from build123d import *
from OCP.BRepFilletAPI import BRepFilletAPI_MakeChamfer

# Parameters (mm, degrees)
SKETCH1_W                = 13.2
SKETCH1_H                = 8
BOSS_EXTRUDE1_DEPTH      = 2
CUT_EXTRUDE1_DEPTH       = 12.914696807
CUT_EXTRUDE1_DEPTH_BACK  = 12.914696807
SKETCH3_W                = 2
SKETCH3_H                = 8
BOSS_EXTRUDE2_DEPTH      = 3.65
BOSS_EXTRUDE3_DEPTH      = 2
BOSS_EXTRUDE4_DEPTH      = 1.25
BOSS_EXTRUDE5_DEPTH      = 2.1
BOSS_EXTRUDE6_DEPTH      = 2.25
CHAMFER3_SIZE            = 1.5
CHAMFER4_SIZE            = 0.3
CHAMFER3_OF_MIRROR1_SIZE = 1.5
CHAMFER4_OF_MIRROR1_SIZE = 0.3
CUT_EXTRUDE2_DEPTH       = 15.141428499
CUT_EXTRUDE2_DEPTH_BACK  = 15.141428499
SKETCH10_W               = 1
SKETCH10_H               = 8
CUT_EXTRUDE3_DEPTH       = 15.418477728
CUT_EXTRUDE3_DEPTH_BACK  = 1
SKETCH12_W               = 6
SKETCH12_H               = 3.8
CUT_EXTRUDE4_DEPTH       = 15.418477728
CUT_EXTRUDE5_REACH       = 24.67
SKETCH13_W               = 1.15
SKETCH13_H               = 2.4
CHAMFER7_SIZE            = 0.5
CHAMFER7_SIZE_2          = 0.353553391
CUT_EXTRUDE6_REACH       = 15.658
SKETCH14_W               = 2
SKETCH14_H               = 1.25
CHAMFER8_SIZE            = 0.5


with BuildPart() as part:
    # Sketch1 → Boss-Extrude1 (new body)
    with BuildSketch(Plane(origin=(0, 0, 0), x_dir=(1, 0, 0), z_dir=(0, 1, 0))):
        with Locations((-2, 0)):
            Rectangle(SKETCH1_W, SKETCH1_H)
        with BuildLine():
            ThreePointArc((0, 1.2), (-1.2, 0), (0, -1.2))
            ThreePointArc((0, -1.2), (0.848528137, -0.848528137), (1.2, 0))
            ThreePointArc((1.2, 0), (0.848528137, 0.848528137), (0, 1.2))
        make_face(mode=Mode.SUBTRACT)
    extrude(amount=-BOSS_EXTRUDE1_DEPTH)

    # Sketch2 → Cut-Extrude1 (cut, two sides: drawn at the far end of the back side and taken through both)
    with BuildSketch(Plane(origin=(0, 0, -4), x_dir=(-1, 0, 0), z_dir=(0, 0, -1)).offset(-CUT_EXTRUDE1_DEPTH_BACK)):
        Polygon((8.6, -2), (8.6, -0.75), (3.75, -0.75), (2.5, -2), align=None)
    extrude(amount=CUT_EXTRUDE1_DEPTH + CUT_EXTRUDE1_DEPTH_BACK, mode=Mode.SUBTRACT)

    # Sketch3 → Boss-Extrude2 (add)
    with BuildSketch(Plane.XZ.offset(2)):
        with Locations((3.6, 0)):
            Rectangle(SKETCH3_W, SKETCH3_H)
    extrude(amount=BOSS_EXTRUDE2_DEPTH)

    # Sketch4 → Boss-Extrude3 (add)
    with BuildSketch(Plane(origin=(0, -2, 2), x_dir=(1, 0, 0), z_dir=(0, 1, 0))):
        Polygon((-8.6, -8.1), (0.8, -8.1), (2.5, -8.1), (2.5, -2), (0.8, -2), (-8.6, -2), align=None)
    boss_extrude3 = extrude(amount=BOSS_EXTRUDE3_DEPTH)

    # Sketch5 → Boss-Extrude4 (add)
    with BuildSketch(Plane.XZ.offset(2)):
        Polygon((-8.6, 10.1), (-6.6, 10.1), (-1.2, 10.1), (0.8, 10.1), (-1.2, 8.1), (-6.6, 8.1), (-6.6, 4), (-8.6, 4), align=None)
    boss_extrude4 = extrude(amount=BOSS_EXTRUDE4_DEPTH)

    # Sketch6 → Boss-Extrude5 (add)
    with BuildSketch(Plane(origin=(0, 0, 4), x_dir=(-1, 0, 0), z_dir=(0, 0, -1))):
        Polygon((2.5, -2), (2.5, -3.65), (5.4, -0.75), (3.75, -0.75), align=None)
    boss_extrude5 = extrude(amount=BOSS_EXTRUDE5_DEPTH)

    # Sketch8 → Boss-Extrude6 (add)
    with BuildSketch(Plane.XZ.offset(3.25)):
        Polygon((0.8, 10.1), (-1.2, 8.1), (-6, 8.1), (-6, 10.1), align=None)
    boss_extrude6 = extrude(amount=BOSS_EXTRUDE6_DEPTH)

    # Chamfer3
    chamfer3_edges = [part.edges().sort_by_distance(p)[0] for p in [
        (-8.6, -1.625, 10.1),
    ]]
    chamfer(chamfer3_edges, length=CHAMFER3_SIZE)

    # Chamfer4
    chamfer4_edges = [part.edges().sort_by_distance(p)[0] for p in [
        (-6.6, -2.625, 8.1),
    ]]
    chamfer(chamfer4_edges, length=CHAMFER4_SIZE)

    # Mirror1: Boss-Extrude3, Boss-Extrude4, Boss-Extrude5, Boss-Extrude6 across plane
    add(boss_extrude3.mirror(Plane.XY))
    add(boss_extrude4.mirror(Plane.XY))
    add(boss_extrude5.mirror(Plane.XY))
    add(boss_extrude6.mirror(Plane.XY))

    # Chamfer3 of Mirror1
    chamfer3_of_mirror1_edges = [part.edges().sort_by_distance(p)[0] for p in [
        (-8.6, -1.625, -10.1),
    ]]
    chamfer(chamfer3_of_mirror1_edges, length=CHAMFER3_OF_MIRROR1_SIZE)

    # Chamfer4 of Mirror1
    chamfer4_of_mirror1_edges = [part.edges().sort_by_distance(p)[0] for p in [
        (-6.6, -2.625, -8.1),
    ]]
    chamfer(chamfer4_of_mirror1_edges, length=CHAMFER4_OF_MIRROR1_SIZE)

    # Sketch10 → Cut-Extrude2 (cut, two sides: drawn at the far end of the back side and taken through both)
    with BuildSketch(Plane.XZ.offset(0.75).offset(-CUT_EXTRUDE2_DEPTH_BACK)):
        with Locations((-8.1, 0)):
            Rectangle(SKETCH10_W, SKETCH10_H)
    extrude(amount=CUT_EXTRUDE2_DEPTH + CUT_EXTRUDE2_DEPTH_BACK, mode=Mode.SUBTRACT)

    # Sketch11 → Cut-Extrude3 (cut, two sides: drawn at the far end of the back side and taken through both)
    with BuildSketch(Plane(origin=(0, 0, 0), x_dir=(1, 0, 0), z_dir=(0, 1, 0)).offset(-CUT_EXTRUDE3_DEPTH_BACK)):
        Polygon((1.154700538, -2), (-1.154700538, -2), (-1.212435565, -1.9), (-2.309401077, 0), (-1.212435565, 1.9), (-1.154700538, 2), (1.154700538, 2), (2.309401077, 0), align=None)
    extrude(amount=CUT_EXTRUDE3_DEPTH + CUT_EXTRUDE3_DEPTH_BACK, mode=Mode.SUBTRACT)

    # Sketch12 → Cut-Extrude4 (cut, through all)
    with BuildSketch(Plane(origin=(0, 0, 0), x_dir=(1, 0, 0), z_dir=(0, 1, 0))):
        with Locations((-4.6, 0)):
            Rectangle(SKETCH12_W, SKETCH12_H)
    extrude(amount=-CUT_EXTRUDE4_DEPTH, mode=Mode.SUBTRACT)

    # Sketch13 → Cut-Extrude5 (cut, up to next)
    with BuildSketch(Plane.XY.offset(10.1), mode=Mode.PRIVATE) as cut_extrude5_sk1:
        with Locations((0.225, -4.3)):
            Rectangle(SKETCH13_W, SKETCH13_H)
    cut_extrude5_tool1 = extrude(cut_extrude5_sk1.sketch, amount=-CUT_EXTRUDE5_REACH, mode=Mode.PRIVATE) & part.part
    add(cut_extrude5_tool1.solids().sort_by_distance((0.225, -4.3, 10.1))[0], mode=Mode.SUBTRACT)

    # Chamfer7
    chamfer7_edges = [part.edges().sort_by_distance(p)[0] for p in [
        (-1.6, -1, 1.9),
        (-1.6, -1, -1.9),
    ]]
    chamfer(chamfer7_edges, length=CHAMFER7_SIZE)
    chamfer7_2_edges_1 = [part.edges().sort_by_distance(p)[0] for p in [
        (-6.6, -3.25, -5.9),
        (-6.45, -3.25, -7.95),
        (-6.15, -3.25, -8.1),
        (-6.15, -3.25, 8.1),
        (-6.45, -3.25, 7.95),
        (-6.6, -3.25, 5.9),
        (-8.6, -3.25, 6.3),
        (-7.85, -3.25, 9.35),
        (-6.55, -3.25, 10.1),
        (-6, -4.375, 10.1),
        (-6, -4.375, -10.1),
        (-6.55, -3.25, -10.1),
        (-7.85, -3.25, -9.35),
        (-8.6, -3.25, -6.3),
        (-3.6, -5.5, 8.1),
        (-0.775, -5.5, 8.525),
        (-0.2, -5.5, -9.1),
        (-3.6, -5.5, -8.1),
        (2.6, -3.825, 4),
        (2.6, -3.825, -4),
        (2.6, -5.65, 0),
        (-1.377350269, 0, 1.614359354),
        (0, 0, 2),
        (1.732050808, 0, 1),
        (1.732050808, 0, -1),
        (0, 0, -2),
        (-1.377350269, 0, -1.614359354),
        (4.6, -2.825, -4),
        (4.6, -2.825, 4),
        (-8.6, 0, -6.3),
        (-7.85, 0, -9.35),
        (-8.6, 0, 6.3),
        (-7.85, 0, 9.35),
        (-2.3, 0, -10.1),
        (2.5, 0, -7.05),
        (3.55, 0, -4),
        (4.6, 0, 0),
        (3.55, 0, 4),
        (2.5, 0, 7.05),
        (-2.3, 0, 10.1),
        (2.5, -1, -10.1),
        (2.5, -1, 10.1),
        (-6, -4.375, 8.1),
        (-6, -4.375, -8.1),
        (-7.6, -0.75, 2.95),
        (-7.6, -0.75, -2.95),
    ]]
    chamfer7_2_edges_2 = [part.edges().sort_by_distance(p)[0] for p in [
        (-2.5, -3.65, -2.95),
    ]]
    chamfer7_2_side_2 = [part.faces().sort_by_distance(p)[0] for p in [
        (-2.5, -3.642928932, -2.95),
    ]]
    chamfer7_2_edges_3 = [part.edges().sort_by_distance(p)[0] for p in [
        (-2.5, -3.65, 2.95),
    ]]
    chamfer7_2_side_3 = [part.faces().sort_by_distance(p)[0] for p in [
        (-2.5, -3.642928932, 2.95),
    ]]
    chamfer7_2 = BRepFilletAPI_MakeChamfer(part.part.solid().wrapped)
    for e in chamfer7_2_edges_1:
        chamfer7_2.Add(CHAMFER7_SIZE, e.wrapped)
    for e in chamfer7_2_edges_2:
        chamfer7_2.Add(CHAMFER7_SIZE_2, CHAMFER7_SIZE, e.wrapped, chamfer7_2_side_2[0].wrapped)
    for e in chamfer7_2_edges_3:
        chamfer7_2.Add(CHAMFER7_SIZE_2, CHAMFER7_SIZE, e.wrapped, chamfer7_2_side_3[0].wrapped)
    add(Compound.cast(chamfer7_2.Shape()), mode=Mode.REPLACE)

    # Cut-Extrude6: up to this face of the body (flat: up to its plane)
    cut_extrude6_end = Plane(part.part.faces().sort_by_distance((1.4, -2, 9.875917426))[0])
    # Sketch14 → Cut-Extrude6 (cut, up to the picked face)
    with BuildSketch(Plane.XZ.offset(3.25), mode=Mode.PRIVATE) as cut_extrude6_sk1:
        with Locations((-7.6, -6.1)):
            Rectangle(SKETCH14_W, SKETCH14_H)
    cut_extrude6_tool1 = split(extrude(cut_extrude6_sk1.sketch, amount=-CUT_EXTRUDE6_REACH, mode=Mode.PRIVATE), bisect_by=cut_extrude6_end, keep=Keep.BOTH, mode=Mode.PRIVATE)
    # Sketch14 → Cut-Extrude6 (cut, up to the picked face)
    with BuildSketch(Plane.XZ.offset(3.25), mode=Mode.PRIVATE) as cut_extrude6_sk2:
        with Locations((-7.6, 6.1)):
            Rectangle(SKETCH14_W, SKETCH14_H)
    cut_extrude6_tool2 = split(extrude(cut_extrude6_sk2.sketch, amount=-CUT_EXTRUDE6_REACH, mode=Mode.PRIVATE), bisect_by=cut_extrude6_end, keep=Keep.BOTH, mode=Mode.PRIVATE)
    add(cut_extrude6_tool1.solids().sort_by(Axis((-7.6, -3.25, -6.1), (0, 1, 0)))[0], mode=Mode.SUBTRACT)
    add(cut_extrude6_tool2.solids().sort_by(Axis((-7.6, -3.25, 6.1), (0, 1, 0)))[0], mode=Mode.SUBTRACT)

    # Chamfer8
    chamfer8_edges = [part.edges().sort_by_distance(p)[0] for p in [
        (-8.6, -2, -6.1),
        (-8.6, -2, 6.1),
    ]]
    chamfer(chamfer8_edges, length=CHAMFER8_SIZE)


solid = part.part
Input: part model. Units: mm. Frame: model coordinates. A direction names the side the tool comes from. Give positions to 0.01 mm unless a question says otherwise; leave off trailing zeros. Loops run counter-clockwise (first coordinate to the right, second up) from the corner with the lowest first, then second, coordinate; pieces in that order, holes last. Notation, with made-up numbers: (-3, 83) -> (48, 83) arc R24 cw to (48, 107) -> close; hole circle Ø9 at (41, -9). An arc over 180 degrees is marked (long way). Answer as a JSON object with one key per item and string values. Group by question number.
Item 1: Cut plane D-D, the plane x = 3.75. Return the cut outline in (y, z), and give its area (4 significant figures).
Item 2: Pull-direction query (Z, two-part tool) for faces 4 (the flat face through (-3, -5.5, 9)), 5 (the flat face through (-4, -1, -1.9)), 6 (the flat face through (-7.665, -0.254, 9.186)); classes: released by +Z, released by -Z, zero draft, split by the parting line, or undercut.
Item 3: Cut plane A-A, the plane x = -3.75. Return the cut outline in (y, z), and give its area (3 significant figures).
Item 4: Line query: probe 1 along Z at (x, y) = (-1.75, -4.2); probe 2 along Z at (x, y) = (-8, -2.9) (3 decimals); probe 3 along X at (y, z) = (-1.25, 1.25). Output: solid intervals per line, ascending.
Item 5: Pin query (flat end, axial travel): P1, Ø0.5, axis at x = 3.5, y = -2.5, coming from the -Z side; P2, Ø2, axis at y = -0.5, z = 5.5, coming from the +X side; P3, Ø0.6, axis at y = -4.5, z = 9.5, coming from the +X side; P4, Ø1.4, axis at x = -7.5, y = -2.5, coming from the -Z side. Return the tip coordinate at first contact, or that it passes through.
Item 6: Cut plane C-C, the plane z = 4.5. Return the cut outline in (x, y), and give its area (3 significant figures).
Item 7: Reachability of faces 1 (the flat face through (1.96, -0.25, 1.11)), 2 (the flat face through (-3.1, -2.5, -4)), 3 (the flat face through (-4.11, -2.04, -2.96)) from +Z, -Z, +X, -X, +Y, -Y: full face, straight path, thin tool, end or side. Return the list, or none.
Item 8: Cut plane B-B, the plane y = -3.6. Return the cut outline in (x, z).
Checks:
{
 "1": {"outline": "(-5.65, -4) -> (-0.5, -4) -> (0, -3.5) -> (0, 3.5) -> (-0.5, 4) -> (-5.65, 4) -> close", "area": "44.95 mm²"},
 "2": {"face 4": "zero draft", "face 5": "undercut", "face 6": "released by +Z"},
 "3": {"outline": "(-5.5, -10.1) -> (-0.5, -10.1) -> (0, -9.6) -> (0, -1.9) -> (-2.4, -1.9) -> (-2.4, -4) -> (-2, -4) -> (-2, -8.1) -> (-5, -8.1) -> (-5.5, -8.6) -> close; (-5.5, 8.6) -> (-5, 8.1) -> (-2, 8.1) -> (-2, 4) -> (-2.4, 4) -> (-2.4, 1.9) -> (0, 1.9) -> (0, 9.6) -> (-0.5, 10.1) -> (-5.5, 10.1) -> close", "area": "48.0 mm²"},
 "4": {"probe 1": "z = -10.1 to -8.1, 8.1 to 10.1", "probe 2": "z = -8.988 to -6.725, -5.475 to -4, 4 to 5.475, 6.725 to 8.988", "probe 3": "x = -1.6 to 4.6"},
 "5": {"P1": "stops at z = -4", "P2": "stops at x = 2.5", "P3": "stops at x = -0.35", "P4": "stops at z = -10.1"},
 "6": {"outline": "(-8.6, -2.75) -> (-8.1, -3.25) -> (-7.1, -3.25) -> (-6.6, -2.75) -> (-6.6, -2) -> (2.5, -2) -> (2.5, -0.5) -> (2, 0) -> (-8.1, 0) -> (-8.6, -0.5) -> close", "area": "24.2 mm²"},
 "7": {"face 1": "+Y", "face 2": "+X, -Y", "face 3": "-X, -Y"},
 "8": {"outline": "(-6, -9.6) -> (-5.5, -10.1) -> (0.8, -10.1) -> (-1.2, -8.1) -> (-5.5, -8.1) -> (-6, -8.6) -> close; (-6, 8.6) -> (-5.5, 8.1) -> (-1.2, 8.1) -> (-0.35, 8.95) -> (-0.35, 10.1) -> (-5.5, 10.1) -> (-6, 9.6) -> close; (2.6, -3.5) -> (3.1, -4) -> (4.1, -4) -> (4.6, -3.5) -> (4.6, 3.5) -> (4.1, 4) -> (3.1, 4) -> (2.6, 3.5) -> close"}
}
